Geometry: final body of the model. Coordinates: model frame, mm. Face numbers are marked on the shaded views. A direction names the side the tool comes from. Coordinates: 2 decimals unless noted, no trailing zeros. Write each loop counter-clockwise with the first axis right and the second up, starting at its lowest first coordinate (ties: lowest second). Pieces come first, ordered by that corner, then holes. Notation, with made-up numbers: (-33, 38.5) - (-23, 38.5) arc R29 cw to (-23, 64.5) - close; hole circle Ø6 at (25.5, 15.5). An arc over 180 degrees is marked (long way). Put each result on its own line as item: value.
```python
from build123d import *

# Parameters (mm, degrees)
SKETCH2_W           = 10.5
SKETCH2_H           = 10
BOSS_EXTRUDE1_DEPTH = 2
SKETCH3_W           = 2
SKETCH3_H           = 10
BOSS_EXTRUDE2_DEPTH = 2
SKETCH4_W           = 2
SKETCH4_H           = 10
BOSS_EXTRUDE3_DEPTH = 10.5
SKETCH18_W          = 2
SKETCH18_H          = 10
BOSS_EXTRUDE6_DEPTH = 19
SKETCH19_W          = 8.99
SKETCH19_H          = 5
CUT_EXTRUDE1_DEPTH  = 19
SKETCH20_W          = 2
SKETCH20_H          = 10
BOSS_EXTRUDE7_DEPTH = 19
SKETCH21_W          = 8.99
SKETCH21_H          = 5
CUT_EXTRUDE2_DEPTH  = 19
BOSS_EXTRUDE8_REACH = 54.114
SKETCH22_W          = 5
SKETCH22_H          = 5
SKETCH23_W          = 5
SKETCH23_H          = 5
BOSS_EXTRUDE9_DEPTH = 10
LOFT1_DEPTH         = 7
LOFT1_DRAFT         = 4.0856168


# Read off the part's stored shape, not the designer's step: Loft1
with BuildPart() as part:
    # Sketch2 → Boss-Extrude1 (new body)
    with BuildSketch(Plane.XY):
        with Locations((5.25, -15)):
            Rectangle(SKETCH2_W, SKETCH2_H)
    extrude(amount=BOSS_EXTRUDE1_DEPTH)

    # Sketch3 → Boss-Extrude2 (add)
    with BuildSketch(Plane(origin=(10.5, 0, 0), x_dir=(0, 0, -1), z_dir=(1, 0, 0))):
        with Locations((-1, -15)):
            Rectangle(SKETCH3_W, SKETCH3_H)
    extrude(amount=BOSS_EXTRUDE2_DEPTH)

    # Sketch4 → Boss-Extrude3 (add)
    with BuildSketch(Plane(origin=(0, 0, 0), x_dir=(-1, 0, 0), z_dir=(0, 0, -1))):
        with Locations((-11.5, -15)):
            Rectangle(SKETCH4_W, SKETCH4_H)
    extrude(amount=BOSS_EXTRUDE3_DEPTH)

    # Sketch18 → Boss-Extrude6 (add)
    with BuildSketch(Plane(origin=(0, 0, -10.5), x_dir=(-1, 0, 0), z_dir=(0, 0, -1))):
        with Locations((-11.5, -15)):
            Rectangle(SKETCH18_W, SKETCH18_H)
    extrude(amount=BOSS_EXTRUDE6_DEPTH)

    # Sketch19 → Cut-Extrude1 (cut)
    with BuildSketch(Plane(origin=(12.5, 0, 0), x_dir=(0, 0, -1), z_dir=(1, 0, 0))):
        with Locations((15.005, -11.5)):
            Rectangle(SKETCH19_W, SKETCH19_H)
    extrude(amount=-CUT_EXTRUDE1_DEPTH, mode=Mode.SUBTRACT)

    # Sketch20 → Boss-Extrude7 (add)
    with BuildSketch(Plane.ZY):
        with Locations((1, -15)):
            Rectangle(SKETCH20_W, SKETCH20_H)
    extrude(amount=BOSS_EXTRUDE7_DEPTH)

    # Sketch21 → Cut-Extrude2 (cut)
    with BuildSketch(Plane.XY.offset(2)):
        with Locations((-4.505, -11.5)):
            Rectangle(SKETCH21_W, SKETCH21_H)
    extrude(amount=-CUT_EXTRUDE2_DEPTH, mode=Mode.SUBTRACT)

    # Sketch22 → Boss-Extrude8 (add, up to next)
    with BuildSketch(Plane(origin=(9.371320344, 0, 9.371320344), x_dir=(0.7071067811865476, 0, -0.7071067811865476), z_dir=(0.7071067811865476, 0, 0.7071067811865476)), mode=Mode.PRIVATE) as boss_extrude8_sk1:
        with Locations((7.424621202, -17.5)):
            Rectangle(SKETCH22_W, SKETCH22_H)
    boss_extrude8_tool1 = extrude(boss_extrude8_sk1.sketch, amount=-BOSS_EXTRUDE8_REACH, mode=Mode.PRIVATE) - part.part
    add(boss_extrude8_tool1.solids().sort_by_distance((14.62132, -17.5, 4.12132))[0])

    # Sketch23 → Boss-Extrude9 (add)
    with BuildSketch(Plane(origin=(9.371320344, 0, 9.371320344), x_dir=(0.7071067811865475, 0, -0.7071067811865476), z_dir=(0.7071067811865476, 0, 0.7071067811865475))):
        with Locations((7.424621202, -17.5)):
            Rectangle(SKETCH23_W, SKETCH23_H)
    extrude(amount=BOSS_EXTRUDE9_DEPTH)


with BuildPart() as loft1_tool:
    # Loft1 outline → Loft1 (with draft: the straight prism first)
    with BuildSketch(Plane(origin=(0, -8, 0), x_dir=(1, 0, 0), z_dir=(0, 1, 0))):
        Polygon((17.096194078, -9.424621202), (19.924621202, -12.253048327), (22.753048327, -9.424621202), (19.924621202, -6.596194078), align=None)
    extrude(amount=-LOFT1_DEPTH)
    # Loft1: the draft: its side faces are tilted about the plane it starts from
    loft1_sides = [loft1_tool.faces().sort_by_distance(p)[0] for p in [
        (18.51040764, -11.5, 10.838834765),
        (21.338834764, -11.5, 10.838834764),
        (21.338834764, -11.5, 8.01040764),
        (18.51040764, -11.5, 8.01040764),
    ]]
    draft(loft1_sides, Plane(origin=(0, -8, 0), x_dir=(1, 0, 0), z_dir=(0, 1, 0)), LOFT1_DRAFT)


with BuildPart() as part_1:
    add(part.part)

    # Loft1: add loft1_tool
    add(loft1_tool.part)


solid = part_1.part
```
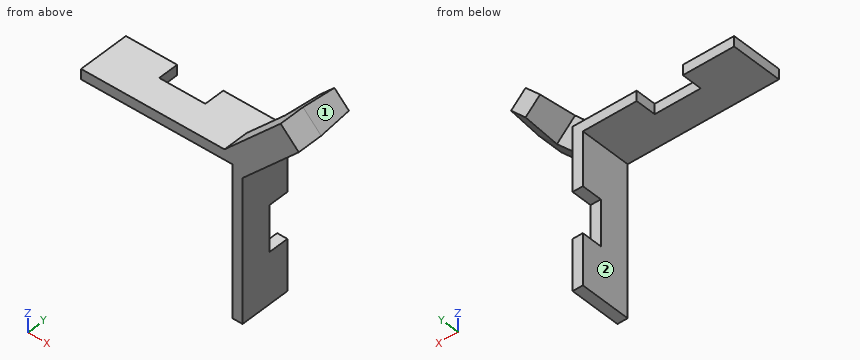
1. Set-up query: the marked faces 1 and 2. Return all of +Z, -Z, +X, -X, +Y, -Y with unobstructed straight access to the full face (end or side cutting, diameter ignored); none if empty.
Answer below:
face 1: +Z, +X, +Y
face 2: -Z, -X, +Y, -Y
2. Section query D-D (z = -11.5). Return loops of the section in (x, y), then the cut area to 3 significant figures.
Answer below:
outline: (10.5, -20) - (12.5, -20) - (12.5, -14) - (10.5, -14) - close
area: 12.0 mm²
3. Pin query (flat end, axial travel): pin 1 Ø2 at (y, z) = (-11.5, 0.5) entering from +X; pin 2 Ø1 at (x, z) = (-15, 1) entering from +Y; pin 3 Ø2 at (x, y) = (11, -12.5) entering from +Z. Return the tip coordinate at first contact, or that it passes through.
Answer below:
pin 1: stops at x = 12.5
pin 2: stops at y = -10
pin 3: stops at z = 2
4. Section query A-A (y = -13.5). Return loops of the section in (x, z), then the cut area to 3 significant figures.
Answer below:
outline: (-19, 0) - (-9, 0) - (-9, 2) - (-19, 2) - close; (-0.01, 0) - (10.5, 0) - (10.5, -10.51) - (12.5, -10.51) - (12.5, 2) - (-0.01, 2) - close; (10.5, -29.5) - (12.5, -29.5) - (12.5, -19.5) - (10.5, -19.5) - close; (16.54, 9.42) - (19.92, 6.04) - (23.31, 9.42) - (19.92, 12.81) - close
area: 109 mm²
5. Ray query, probe 1 along Z at (x, y) = (-16.5, -16.25); probe 2 along Y at (x, z) = (12, -2); probe 3 along X at (y, z) = (-13.5, -10). Return the intervals inside material, ascending. Write a range as from..to.
Answer below:
probe 1: z = 0..2
probe 2: y = -20..-10
probe 3: x = 10.5..12.5
6. Section query B-B (y = -16.5). Return loops of the section in (x, z).
Answer below:
outline: (-19, 0) - (10.5, 0) - (10.5, -29.5) - (12.5, -29.5) - (12.5, -1.54) - (23.46, 9.42) - (19.92, 12.96) - (8.96, 2) - (-19, 2) - close
7. Section query C-C (x = 18.5). Return loops of the section in (y, z).
Answer below:
outline: (-20, 4.46) - (-15, 4.46) - (-15, 7.31) - (-8, 8.02) - (-8, 10.83) - (-15, 11.54) - (-20, 11.54) - close
